Autodesk Inventor part; units mm, degrees
ref_plane "YZ Plane" through (0, 0, 0) normal (1, 0, 0) x (0, 1, 0)
ref_plane "XZ Plane" through (0, 0, 0) normal (0, 1, 0) x (-1, 0, 0)
ref_plane "XY Plane" through (0, 0, 0) normal (0, 0, 1) x (1, 0, 0)
sketch "Sketch1" plane through (0, 0, 0) normal (0, 1, 0) x (-1, 0, 0)
  line L0 (40, 5) -> (40, -39)
  line L1 (0, -39) -> (0, 0)
  line L2 (40, 5) -> (30, 5)
  line L3 (30, 5) -> (30, 11)
  line L4 (30, 11) -> (27, 11)
  line L5 (27, 11) -> (27, 7)
  line L6 (27, -39) -> (27, -45)
  line L7 (27, -45) -> (30, -45)
  line L8 (30, -45) -> (30, -39)
  line L9 (30, 5) -> (40, 5)
  line L10 (40, -39) -> (30, -39)
  line L11 (27, -39) -> (0, -39)
  line L12 (0, 3) -> (0, 0)
  line L13 (0, 5) -> (0, 3)
  line L14 (27, 5) -> (0, 5)
  line L15 (27, 7) -> (27, 5)
  dimension "d0" = 40
  dimension "d1" = 44
  dimension "d2" = 10
  dimension "d3" = 6
  dimension "d4" = 3
  dimension "d5" = 6
extrude "Extrusion1" add sketch "Sketch1" along normal blind 20
sketch "Sketch2" plane through (-30, 0, 5) normal (-1, 0, 0) x (0, 0, 1)
  line L0 (6, 0) -> (6, 20)
  line L1 (6, 10) -> (3, 10)
  line L2 (3, 10) -> (3, 15)
  line L3 (3, 15) -> (3, 5)
  circle A0 centre (3, 15) radius 1.5
  circle A1 centre (3, 5) radius 1.5
  circle A2 centre (-42, 15) radius 1.5
  circle A3 centre (-42, 5) radius 1.5
  dimension "d8" = 5
  dimension "d9" = 10
  dimension "d10" = 3
  dimension "d11" = 3
  dimension "d12" = 3
  dimension "d13" = 3
extrude "Extrusion2" cut sketch "Sketch2" against normal blind 20
sketch "Sketch3" plane through (-40, 0, -39) normal (-1, 0, 0) x (0, 0, 1)
  line L0 (0, 0) -> (0, 20)
  line L1 (0, 10) -> (10, 10)
  circle A0 centre (10, 10) radius 3
  dimension "d16" = 10
  dimension "d17" = 6
extrude "Extrusion3" add sketch "Sketch3" along normal blind 4
sketch "Sketch4" plane through (0, 0, 0) normal (1, 0, 0) x (0, 0, -1)
  line L0 (-5, 0) -> (39, 0)
  line L1 (39, 0) -> (39, 20)
  line L2 (-5, 20) -> (39, 20)
  line L3 (0, 0) -> (0, 20)
extrude "Extrusion4" cut sketch "Sketch4" against normal blind 2
sketch "Sketch5" plane through (0, 0, 0) normal (0, -1, 0) x (1, 0, 0)
  line L0 (-2, 0) -> (0, 0)
  line L1 (0, 0) -> (0, -39)
  line L2 (0, -39) -> (-2, -39)
  line L3 (-2, -39) -> (-2, 0)
extrude "Extrusion5" add sketch "Sketch5" against normal up to surface (20 mm away)
sketch "Sketch6" plane through (0, 0, 5) normal (1, 0, 0) x (0, 0, -1)
  line L0 (44, 20) -> (0, 20)
  line L1 (0, 0) -> (0, 20)
  line L2 (44, 0) -> (0, 0)
  line L3 (44, 0) -> (44, 20)
  point P0 (5, 0)
extrude "Extrusion6" cut sketch "Sketch6" against normal blind 2
properties part number "Elbow Servo"
Input: part model. Units: mm. Frame: model coordinates. A direction names the side the tool comes from. Round coordinates to 2 decimals unless told otherwise and drop trailing zeros. Loops run counter-clockwise (first coordinate to the right, second up) from the corner with the lowest first, then second, coordinate; pieces in that order, holes last. Notation, with made-up numbers: M 76.25,62 L 86.25,62 A18 cw 86.25,87 Z; hole C 31,60 d8. An arc over 180 degrees is marked long. Answer in a Markdown table with one row per item. Add a question column.
1. Set-up query: faces 5 (the face through (-30, 15, -37)), 6 (the face through (-27, 10, -42)), 7 (the face through (-35, 10, 5)), 8 (the face through (-15, 10, 5)), 9 (the face through (-30, 10, -42)). Return all of +Z, -Z, +X, -X, +Y, -Y with unobstructed straight access to the full face (end or side cutting, diameter ignored); none if empty.
2. Ray query, probe 1 along Y at (x, z) = (-17.5, -37); probe 2 along Z at (x, y) = (-37.5, 11.5); probe 3 along X at (y, z) = (6.5, -27.5). Return the intervals inside material, ascending.
3. Contact query for flat-ended pins moving along their axis: pin 1 (1 mm diameter, centred on x = -32.5, y = 13.5, fed in from -Z); pin 2 (2.5 mm diameter, centred on y = 4.5, z = -37, fed in from -X); pin 3 (5 mm diameter, centred on y = 15, z = 8, fed in from +X). Output: stop coordinate, or through.
4. Section A-A (y = 5). Output: boundary loops of the cut face in (x, z).
5. Section B-B (z = 8). Output: boundary loops of the cut face in (x, y), and give its area (3 significant figures).
6. Section C-C (z = -37). Output: boundary loops of the cut face in (x, y).
7. Mould query, pull axis Z, two halves, no side actions, for faces 1 (the face through (-14, 10, -39)), 2 (the face through (-20.1, 4.1, -38.2)), 3 (the face through (-2, 10, -17)), 4 (the face through (-20.1, 14.1, -38.2)). Classes: released by +Z, released by -Z, zero draft, split by the parting line, or undercut.
8. Section D-D (x = -23.5). Output: boundary loops of the cut face in (y, z).
Values follow:
| question | item | result |
|---|---|---|
| 1 | face 5 | none |
| 1 | face 6 | -Z, +X, +Y, -Y |
| 1 | face 7 | +Z, -X, +Y, -Y |
| 1 | face 8 | +Z, +X, +Y, -Y |
| 1 | face 9 | -Z, -X, +Y, -Y |
| 2 | probe 1 | 0 to 3.5, 6.5 to 13.5, 16.5 to 20 |
| 2 | probe 2 | -39 to 5 |
| 2 | probe 3 | -40 to -2 |
| 3 | pin 1 | z = -39 |
| 3 | pin 2 | x = -40 |
| 3 | pin 3 | x = -27 |
| 4 | outline | M -40,-39 L -30,-39 L -30,-45 L -27,-45 L -27,-39 L -2,-39 L -2,5 L -27,5 L -27,6.5 L -30,6.5 L -30,5 L -40,5 Z; M -30,9.5 L -27,9.5 L -27,11 L -30,11 Z; hole M -30,-38.5 L -10,-38.5 L -10,-35.5 L -30,-35.5 Z |
| 5 | outline | M -30,0 L -27,0 L -27,3.5 L -30,3.5 Z; M -30,6.5 L -27,6.5 L -27,13.5 L -30,13.5 Z; M -30,16.5 L -27,16.5 L -27,20 L -30,20 Z |
| 5 | area | 42.0 mm^2 |
| 6 | outline | M -40,0 L -2,0 L -2,20 L -40,20 Z; hole M -30,3.5 L -10,3.5 L -10,6.5 L -30,6.5 Z; hole M -30,13.5 L -10,13.5 L -10,16.5 L -30,16.5 Z |
| 7 | face 1 | released by -Z |
| 7 | face 2 | undercut |
| 7 | face 3 | zero draft |
| 7 | face 4 | undercut |
| 8 | outline | M 0,-39 L 20,-39 L 20,5 L 0,5 Z; hole C 5,-37 d3; hole C 15,-37 d3 |
